CAD build for the part. Positions are in the model's coordinates, mm. A direction names the side the tool comes from. Give positions to 0.01 mm unless a question says otherwise; leave off trailing zeros. Loops run counter-clockwise (first coordinate to the right, second up) from the corner with the lowest first, then second, coordinate; pieces in that order, holes last.
Item 1: Saw through at B-B on x = 81.5. Give the cut face in (y, z).
Item 2: Mould opens along X. For faces 1 (the cylindrical face through (96.45, 23.5, 75.13)), 2 (the flat face through (4.744, 38.633, 75.133)), 3 (the flat face through (38, 12.7, 75)), 4 (the flat face through (48.4, 21.7, 152.4)) say: released by +X, released by -X, zero draft, split by the parting line, or undercut.
Item 3: Drop flat-ended pins along their axis: P1, Ø7, axis at x = 37, z = 53.5, coming from the +Y side; P2, Ø1, axis at y = 20.5, z = 66, coming from the +X side; P3, Ø12, axis at y = 68, z = 63, coming from the -X side; P4, Ø2, axis at x = 21, y = 23, coming from the -Z side. Give the stop position or say it passes through.
Item 4: Probe probe 1 along Y at (x, z) = (91.5, 23); probe 2 along Y at (x, z) = (37.5, 129); probe 3 along X at (y, z) = (19, 73.5). List the from-to ranges inside material, lowest first.
Item 5: Which spindle directions (+Z, -Z, +X, -X, +Y, -Y) get a long thin tool onto all of the face, cutting with end or side? Do faces 5 (the flat face through (48.4, 21.7, 0)), 6 (the flat face through (22.056, 50, 75)), 7 (the cylindrical face through (25.9, 16.3, 75.1)). Say none if no direction does.
Item 6: Saw through at A-A on z = 93.5. Give the cut face in (x, y), plus the area to 3 significant figures.
Item 7: Saw through at C-C on y = 33. Give the cut face in (x, z).
from build123d import *

# Parameters (mm, degrees)
BOSS_EXTRUDE1_DEPTH = 152.4


with BuildPart() as part:
    # Sketch1 → Boss-Extrude1 (new body)
    with BuildSketch(Plane.XY):
        with BuildLine():
            Line((0, 0), (98.256183541, 0))
            Line((98.256183541, 0), (98.256183541, 12.7))
            Line((98.256183541, 12.7), (98.256183541, 19.0754))
            ThreePointArc((98.256183541, 19.0754), (96.403751089, 23.547567548), (91.931583541, 25.4))
            Line((91.931583541, 25.4), (53.780783541, 25.4))
            ThreePointArc((53.780783541, 25.4), (49.308615993, 23.547567548), (47.456183541, 19.0754))
            Line((47.456183541, 19.0754), (47.456183541, 19.0246))
            ThreePointArc((47.456183541, 19.0246), (45.603751089, 14.552432452), (41.131583541, 12.7))
            Line((41.131583541, 12.7), (34.756183541, 12.7))
            ThreePointArc((34.756183541, 12.7), (25.77592742, 16.419743879), (22.056183541, 25.4))
            Line((22.056183541, 25.4), (22.056183541, 76.2))
            Line((22.056183541, 76.2), (9.356183541, 76.2))
            Line((9.356183541, 76.2), (0, 0))
        make_face()
    extrude(amount=BOSS_EXTRUDE1_DEPTH)


solid = part.part
Results below:
1. outline: (0, 0) - (25.4, 0) - (25.4, 152.4) - (0, 152.4) - close
2. face 1: released by +X
2. face 2: released by -X
2. face 3: undercut
2. face 4: zero draft
3. P1: stops at y = 12.76
3. P2: stops at x = 98.19
3. P3: stops at x = 7.61
3. P4: stops at z = 0
4. probe 1: y = 0 to 25.4
4. probe 2: y = 0 to 12.7
4. probe 3: x = 2.33 to 23.79, 47.46 to 98.26
5. face 5: -Z, +X, -X, +Y, -Y
5. face 6: +Z, -Z, +X, +Y
5. face 7: +Z, -Z, +Y
6. outline: (0, 0) - (98.26, 0) - (98.26, 19.08) arc R6.32 ccw to (91.93, 25.4) - (53.78, 25.4) arc R6.32 ccw to (47.46, 19.08) - (47.46, 19.02) arc R6.32 cw to (41.13, 12.7) - (34.76, 12.7) arc R12.7 cw to (22.06, 25.4) - (22.06, 76.2) - (9.36, 76.2) - close
6. area: 2,960 mm2
7. outline: (4.05, 0) - (22.06, 0) - (22.06, 152.4) - (4.05, 152.4) - close
